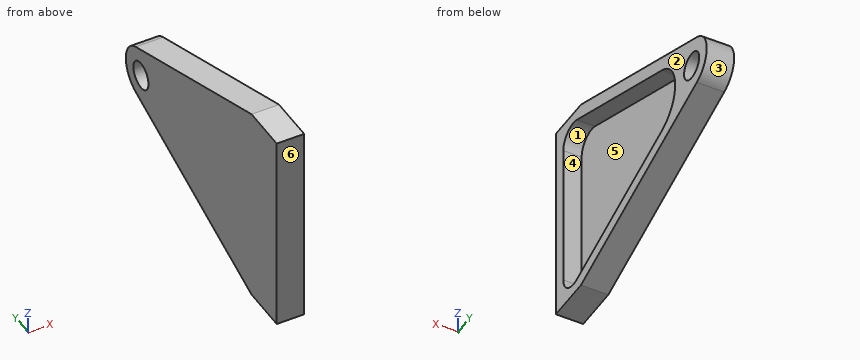
Autodesk Inventor part; units mm, degrees
ref_plane "YZ Plane" through (0, 0, 0) normal (1, 0, 0) x (0, 1, 0)
ref_plane "XZ Plane" through (0, 0, 0) normal (0, 1, 0) x (-1, 0, 0)
ref_plane "XY Plane" through (0, 0, 0) normal (0, 0, 1) x (1, 0, 0)
sketch "Sketch1" plane through (0, 0, 0) normal (1, 0, 0) x (0, 1, 0)
  line L0 (0, 22.5) -> (0, -22.5)
  arc A0 (56.0629, -5.6342) -> (56.0629, 5.6342) centre (54, 0) ccw
  line L1 (0, 22.5) -> (10, 22.5)
  line L2 (0, -22.5) -> (10, -22.5)
  line L3 (10, -22.5) -> (56.0629, -5.6342)
  line L4 (10, 22.5) -> (56.0629, 5.6342)
  point P0 (0, 0)
  dimension "d1" = 6
  dimension "d2" = 10
  dimension "d3" = 54
  dimension "d4" = 45
extrude "Extrusion1" add sketch "Sketch1" along normal blind 6
sketch "Sketch2" plane through (6, 0, 0) normal (1, 0, 0) x (0, 0, -1)
  line L0 (-22.5, 0) -> (22.5, 0)
  line L1 (22.5, 10) -> (5.6342, 56.0629)
  line L2 (-5.6342, 56.0629) -> (-22.5, 10)
  line L3 (-7.5123, 42.2083) -> (-19.9001, 8.3753)
  line L4 (-16.144, 3) -> (16.144, 3)
  line L5 (19.9001, 8.3753) -> (7.5123, 42.2083)
  arc A0 (7.5123, 42.2083) -> (-7.5123, 42.2083) centre (0, 39.4577) ccw
  arc A1 (-19.9001, 8.3753) -> (-16.144, 3) centre (-16.144, 7) ccw
  arc A2 (16.144, 3) -> (19.9001, 8.3753) centre (16.144, 7) ccw
  point P0 (0, 0)
  dimension "d8" = 4
  dimension "d9" = 8
  dimension "d10" = 3
  dimension "d11" = 3
  dimension "d12" = 3
extrude "Extrusion2" cut sketch "Sketch2" against normal blind 4
sketch "Sketch3" plane through (6, 0, 0) normal (1, 0, 0) x (0, 0, -1)
  arc A0 (5.6342, 56.0629) -> (-5.6342, 56.0629) centre (0, 54) ccw
  point P0 (0, 0)
hole "Hole1" at (6, 54, 0) direction (-1, 0, 0) diameter 6 end through all
properties part number "Bearing Short"
Could you check a few things on this model? Use its own coordinates, in mm. Face numbers are marked on the shaded views. A direction names the side the tool comes from. Round coordinates to 2 decimals unless told otherwise and drop trailing zeros. Order: outer loops, then holes, each group sorted by start corner. A loop starts at its lowest first (then second) coordinate and runs counter-clockwise, first axis right, second up.
(1) Imagine slicing it at B-B (z = 0). Write out the boundary of the cut face in (x, y), plus the area to 3 significant figures.
Response values:
outline: (0, 0) - (6, 0) - (6, 3) - (2, 3) - (2, 47.46) - (6, 47.46) - (6, 51) - (0, 51) - close; (0, 57) - (6, 57) - (6, 60) - (0, 60) - close
area: 146 mm2
(2) If we mould it in two halves opening along Y, with no side actions, what happens to the marked faces 1, 2, 3 and 4? For each: released by +Y, released by -Y, zero draft, split by the parting line, or undercut.
Response values:
face 1: undercut
face 2: zero draft
face 3: released by +Y
face 4: undercut
(3) Imagine slicing it at C-C (x = 1.3). Write out the boundary of the cut face in (y, z), plus the area to 3 significant figures.
Response values:
outline: (0, -22.5) - (10, -22.5) - (56.06, -5.63) arc R6 ccw to (56.06, 5.63) - (10, 22.5) - (0, 22.5) - close; hole circle Ø6 at (54, 0)
area: 1,750 mm2
(4) Please list where these lines run through material, in increasing order: line 1 along Y through (x, z) = (1.3, 0); line 2 along Z through (x, y) = (3.9, 54); line 3 along Z through (x, y) = (2.3, 30).
Response values:
line 1: y = 0 to 51, 57 to 60
line 2: z = -6.39 to -3, 3 to 6.39
line 3: z = -15.18 to -11.98, 11.98 to 15.18
(5) Which directions (+Z, -Z, +X, -X, +Y, -Y) give clear straight access to the entire face, cutting with the end or side of a thin tool? Please do the marked faces 5 and 6.
Response values:
face 5: +X
face 6: +Z, -Z, +X, -X, -Y
(6) Imagine slicing it at A-A (x = 3.95). Write out the boundary of the cut face in (y, z), plus the area to 3 significant figures.
Response values:
outline: (0, -22.5) - (10, -22.5) - (56.06, -5.63) arc R6 ccw to (56.06, 5.63) - (10, 22.5) - (0, 22.5) - close; hole (3, -16.14) arc R4 ccw to (8.38, -19.9) - (42.21, -7.51) arc R8 ccw to (42.21, 7.51) - (8.38, 19.9) arc R4 ccw to (3, 16.14) - close; hole circle Ø6 at (54, 0)
area: 556 mm2
(7) Imagine slicing it at D-D (y = 54). Write out the boundary of the cut face in (x, z).
Response values:
outline: (0, -6.39) - (6, -6.39) - (6, -3) - (0, -3) - close; (0, 3) - (6, 3) - (6, 6.39) - (0, 6.39) - close
(8) I'm going to push flat-ended pins straight in: pin 1 (1 mm diameter, centred on x = 1.5, y = 45.5, fed in from -Z); pin 2 (1.2 mm diameter, centred on x = 3.5, z = -1, fed in from +Y); pin 3 (3 mm diameter, centred on y = 50, z = -9.5, fed in from +X). Where does each tip first touch, or does it pass through?
Response values:
pin 1: stops at z = -9.68
pin 2: stops at y = 59.99
pin 3: passes through
